The model under review builds one solid part; all positions refer to its coordinate system, in mm. Face numbers are marked on the shaded views. A direction names the side the tool comes from. Give positions to 0.01 mm unless a question says otherwise; leave off trailing zeros. Order: outer loops, then holes, each group sorted by start corner. A loop starts at its lowest first (then second) coordinate and runs counter-clockwise, first axis right, second up. Notation, with made-up numbers: (55, 68.5) - (96, 68.5) arc R22 ccw to (96, 97.5) - close; hole circle Ø8 at (-33.75, 80.25). An arc over 180 degrees is marked (long way). Write item = value, one per line. Start each with the question number.
1. Wall thickness on probe 1 along X at (y, z) = (-2.75, 0) (3 decimals); probe 2 along X at (y, z) = (1, 0) (3 decimals); probe 3 along Y at (x, z) = (-26.5, 6.5): over which ranges is each line inside the solid? List them lowest first.
2. We need section B-B, the plane x = 0. Give the boundary of the cut face in (y, z) (3 decimals).
3. Mouldability with a two-part tool opening along Z and no side actions: class the marked faces 3, 4 and 5 as pulls with the +Z half, pulls with the -Z half, needs draft (parallel to the pull), parting line crosses it, or undercut.
4. We need section D-D, the plane z = -25. Give the boundary of the cut face in (x, y).
5. We need section C-C, the plane y = -3. Give the boundary of the cut face in (x, z) (3 decimals).
6. Machinability: for the marked faces 1 and 2, which of the approach directions +Z, -Z, +X, -X, +Y, -Y give a long, thin tool a straight path to every point of the face, cutting with its end or side? Answer none if there is none.
7. For P1, Ø2, axis at x = 24, z = 14.5, coming from the +Y side; P2, Ø1.5, axis at y = -2, z = -14, coming from the -X side, all flat-tipped, find the tip position at first contact; note any pin that passes through.
8. We need section A-A, the plane z = 0. Give the boundary of the cut face in (x, y) (3 decimals).
from build123d import *

# Parameters (mm, degrees)
BANDAID_START                  = 0.053848
SKETCH3_R                      = 30.84068
SKETCH3_R_2                    = 15.875
BANDAID_SOLUTION_THICKER_DEPTH = 0.053848
SKETCH4_R                      = 22.86
SKETCH4_R_2                    = 15.875
LIP_FOR_BEARING_DEPTH          = 1.016
SKETCH5_R                      = 30.84068
SKETCH5_R_2                    = 15.875
BOSS_EXTRUDE1_DEPTH            = 0.57912


with BuildPart() as part:
    # Sketch1 → Revolve1 (revolve)
    with BuildSketch(Plane(origin=(0, 0, 0), x_dir=(0, 0, -1), z_dir=(1, 0, 0))):
        Polygon((-15.875, 2.694084), (-15.875, -5.020818), (-30.84068, -5.020818), (-30.84068, -1.062068), (-29.43479, -1.062068), (-29.43479, 1.477932), (-30.84068, 1.477932), (-30.84068, 2.694084), align=None)
    revolve(axis=Axis((0, 0, 0), (0, -1, 0)))

    # Sketch3 → BandAid Solution thicker (add)
    with BuildSketch(Plane(origin=(0, 2.694084, 0), x_dir=(1, 0, 0), z_dir=(0, 1, 0)).offset(BANDAID_START)):
        with Locations(Location((0, 0, 0), (0, 0, 270))):
            Circle(SKETCH3_R)
        with Locations(Location((0, 0, 0), (0, 0, 270))):
            Circle(SKETCH3_R_2, mode=Mode.SUBTRACT)
    extrude(amount=-BANDAID_SOLUTION_THICKER_DEPTH)

    # Sketch4 → Lip for Bearing (add)
    with BuildSketch(Plane(origin=(0, 2.747932, 0), x_dir=(1, 0, 0), z_dir=(0, 1, 0))):
        with Locations(Location((0, 0, 0), (0, 0, 90))):
            Circle(SKETCH4_R)
        with Locations(Location((0, 0, 0), (0, 0, 270))):
            Circle(SKETCH4_R_2, mode=Mode.SUBTRACT)
    extrude(amount=LIP_FOR_BEARING_DEPTH)

    # Sketch5 → Boss-Extrude1 (add)
    with BuildSketch(Plane.XZ.offset(5.020818)):
        with Locations(Location((0, 0, 0), (0, 0, 90))):
            Circle(SKETCH5_R)
        with Locations(Location((0, 0, 0), (0, 0, 90))):
            Circle(SKETCH5_R_2, mode=Mode.SUBTRACT)
    extrude(amount=BOSS_EXTRUDE1_DEPTH)


solid = part.part
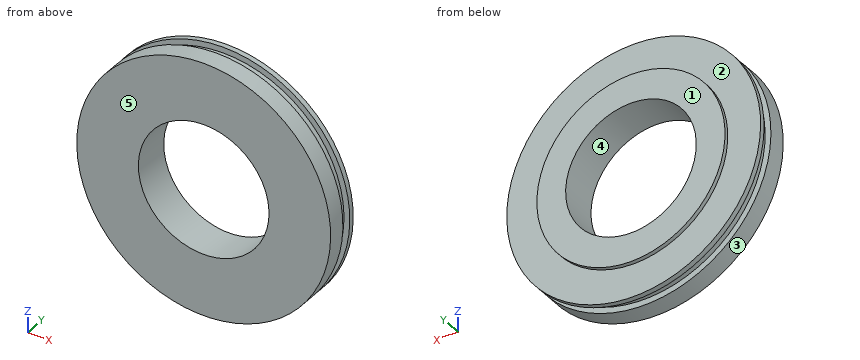
Model answer:
q1.probe_1 = -30.841 to -15.875, 15.875 to 30.841
q1.probe_2 = -29.435 to -15.875, 15.875 to 29.435
q1.probe_3 = -5.6 to 2.75
q2.outline = (-5.6, -30.841) - (-1.062, -30.841) - (-1.062, -29.435) - (1.478, -29.435) - (1.478, -30.841) - (2.748, -30.841) - (2.748, -22.86) - (3.764, -22.86) - (3.764, -15.875) - (-5.6, -15.875) - close; (-5.6, 15.875) - (3.764, 15.875) - (3.764, 22.86) - (2.748, 22.86) - (2.748, 30.841) - (1.478, 30.841) - (1.478, 29.435) - (-1.062, 29.435) - (-1.062, 30.841) - (-5.6, 30.841) - close
q3.face_3 = parting line crosses it
q3.face_4 = undercut
q3.face_5 = needs draft
q4.outline = (-18.06, -5.6) - (18.06, -5.6) - (18.06, -1.06) - (15.54, -1.06) - (15.54, 1.48) - (18.06, 1.48) - (18.06, 2.75) - (-18.06, 2.75) - (-18.06, 1.48) - (-15.54, 1.48) - (-15.54, -1.06) - (-18.06, -1.06) - close
q5.outline = circle Ø61.681 at (0, 0); hole circle Ø31.75 at (0, 0)
q6.face_1 = +Z, -Z, +X, -X, +Y
q6.face_2 = +Y
q7.P1 = 2.75
q7.P2 = -27.85
q8.outline = (-30.841, -5.6) - (-15.875, -5.6) - (-15.875, 3.764) - (-22.86, 3.764) - (-22.86, 2.748) - (-30.841, 2.748) - (-30.841, 1.478) - (-29.435, 1.478) - (-29.435, -1.062) - (-30.841, -1.062) - close; (15.875, -5.6) - (30.841, -5.6) - (30.841, -1.062) - (29.435, -1.062) - (29.435, 1.478) - (30.841, 1.478) - (30.841, 2.748) - (22.86, 2.748) - (22.86, 3.764) - (15.875, 3.764) - close
